from build123d import *

# Parameters (mm, degrees)
SKETCH1_R             = 3.4
SKETCH1_R_2           = 1.9
BOSS_EXTRUDE1_DEPTH   = 5
SKETCH1_R_3           = 14
SKETCH1_R_4           = 10
BOSS_EXTRUDE1_2_DEPTH = 5
BOSS_EXTRUDE3_START   = -5
BOSS_EXTRUDE3_DEPTH   = 5
CUT_EXTRUDE1_DEPTH    = 21.420577857


with BuildPart() as part:
    # Sketch1 → Boss-Extrude1 (new body)
    with BuildSketch(Plane.XY):
        Circle(SKETCH1_R)
        Circle(SKETCH1_R_2, mode=Mode.SUBTRACT)
    extrude(amount=BOSS_EXTRUDE1_DEPTH)



with BuildPart() as body_2:
    # Sketch1 → Boss-Extrude1 2 (new body)
    with BuildSketch(Plane.XY):
        Circle(SKETCH1_R_3)
        Circle(SKETCH1_R_4, mode=Mode.SUBTRACT)
    extrude(amount=BOSS_EXTRUDE1_2_DEPTH)


with BuildPart() as part_1:
    add(part.part)

    add(body_2.part)  # Boss-Extrude3 merges body 2
    # Sketch3 → Boss-Extrude3 (add)
    with BuildSketch(Plane.XY.offset(5).offset(BOSS_EXTRUDE3_START)):
        with BuildLine():
            Line((-2.461082993, -5.681791735), (-1.158545138, -6.104894644))
            ThreePointArc((-1.158545138, -6.104894644), (0.041583332, -6.976727004), (0.5, -8.387490686))
            ThreePointArc((0.5, -8.387490686), (1.026221783, -9.481342425), (2.209302326, -9.752896146))
            ThreePointArc((2.209302326, -9.752896146), (0, -10), (-2.209302326, -9.752896146))
            ThreePointArc((-2.209302326, -9.752896146), (-0.55013353, -8.758786407), (-1.467484664, -7.055976328))
            Line((-1.467484664, -7.055976328), (-2.770022518, -6.632873419))
            ThreePointArc((-2.770022518, -6.632873419), (-4.377477342, -4.842845432), (-3.62455882, -2.557845453))
            ThreePointArc((-3.62455882, -2.557845453), (-3.203111756, -1.874062431), (-3.226850513, -1.071184282))
            ThreePointArc((-3.226850513, -1.071184282), (-2.53927856, -2.260987482), (-1.43690209, -3.081446476))
            ThreePointArc((-1.43690209, -3.081446476), (-3.331173148, -3.837228711), (-2.461082993, -5.681791735))
        make_face()
        with BuildLine():
            Line((-6.164221523, 0.584858813), (-6.164109969, -0.784674291))
            ThreePointArc((-6.164109969, -0.784674291), (-6.622411723, -2.195475308), (-7.822469175, -3.06740542))
            ThreePointArc((-7.822469175, -3.06740542), (-8.700172525, -3.905890853), (-8.592843468, -5.114982027))
            ThreePointArc((-8.592843468, -5.114982027), (-9.510565163, -3.090169944), (-9.958267397, -0.91263928))
            ThreePointArc((-9.958267397, -0.91263928), (-8.500101497, -2.183405771), (-7.164109966, -0.784755745))
            Line((-7.164109966, -0.784755745), (-7.16422152, 0.584777358))
            ThreePointArc((-7.16422152, 0.584777358), (-5.958534597, 2.666706812), (-3.552705858, 2.656742571))
            ThreePointArc((-3.552705858, 2.656742571), (-2.772155254, 2.467223168), (-2.015908439, 2.73790306))
            ThreePointArc((-2.015908439, 2.73790306), (-2.935007106, 1.716313866), (-3.374656916, 0.414355768))
            ThreePointArc((-3.374656916, 0.414355768), (-4.678810484, 1.982365046), (-6.164221523, 0.584858813))
        make_face()
        with BuildLine():
            Line((-1.348615423, 6.04325436), (-2.651084333, 5.619939262))
            ThreePointArc((-2.651084333, 5.619939262), (-4.134458864, 5.619848642), (-5.334551826, 6.491729879))
            ThreePointArc((-5.334551826, 6.491729879), (-6.403224112, 7.067369122), (-7.519971649, 6.591663402))
            ThreePointArc((-7.519971649, 6.591663402), (-5.877852523, 8.090169944), (-3.945245395, 9.188854051))
            ThreePointArc((-3.945245395, 9.188854051), (-4.703218103, 7.409367429), (-2.960178794, 6.570970605))
            Line((-2.960178794, 6.570970605), (-1.657709884, 6.994285702))
            ThreePointArc((-1.657709884, 6.994285702), (0.694900438, 6.490960879), (1.428865848, 4.199802661))
            ThreePointArc((1.428865848, 4.199802661), (1.489825587, 3.398890206), (1.98095058, 2.763301431))
            ThreePointArc((1.98095058, 2.763301431), (0.725344411, 3.321727786), (-0.648750584, 3.337532424))
            ThreePointArc((-0.648750584, 3.337532424), (0.439509241, 5.062397688), (-1.348615423, 6.04325436))
        make_face()
        with BuildLine():
            Line((5.330731354, 3.150077785), (4.525649744, 4.25798777))
            ThreePointArc((4.525649744, 4.25798777), (4.06717562, 5.66873278), (4.525534832, 7.079515131))
            ThreePointArc((4.525534832, 7.079515131), (4.742762387, 8.273765181), (3.945245395, 9.188854051))
            ThreePointArc((3.945245395, 9.188854051), (5.877852523, 8.090169944), (7.519971649, 6.591663402))
            ThreePointArc((7.519971649, 6.591663402), (5.593352853, 6.762646678), (5.334618858, 4.845838918))
            Line((5.334618858, 4.845838918), (6.139700468, 3.737928933))
            ThreePointArc((6.139700468, 3.737928933), (6.388006686, 1.344927632), (4.435793517, -0.06112178))
            ThreePointArc((4.435793517, -0.06112178), (3.692918104, -0.366593497), (3.240203227, -1.030088854))
            ThreePointArc((3.240203227, -1.030088854), (3.383294606, 0.336626808), (2.973707004, 1.648352709))
            ThreePointArc((2.973707004, 1.648352709), (4.950442134, 1.14636879), (5.330731354, 3.150077785))
        make_face()
        with BuildLine():
            Line((4.643188585, -4.096399222), (5.448089696, -2.988358097))
            ThreePointArc((5.448089696, -2.988358097), (6.648111636, -2.116379111), (8.131486169, -2.116348904))
            ThreePointArc((8.131486169, -2.116348904), (9.334412468, -1.953901025), (9.958267397, -0.91263928))
            ThreePointArc((9.958267397, -0.91263928), (9.510565163, -3.090169944), (8.592843468, -5.114982027))
            ThreePointArc((8.592843468, -5.114982027), (8.160100277, -3.229821928), (6.257154566, -3.576077449))
            Line((6.257154566, -3.576077449), (5.452253454, -4.684118574))
            ThreePointArc((5.452253454, -4.684118574), (3.253104814, -5.659749891), (1.312605313, -4.237577998))
            ThreePointArc((1.312605313, -4.237577998), (0.792523319, -3.625457447), (0.021605145, -3.399931355))
            ThreePointArc((0.021605145, -3.399931355), (1.365646649, -3.113680977), (2.486602586, -2.318794424))
            ThreePointArc((2.486602586, -2.318794424), (2.620032257, -4.353902812), (4.643188585, -4.096399222))
        make_face()
    extrude(amount=BOSS_EXTRUDE3_DEPTH)

    # Sketch4 → Cut-Extrude1 (cut, through all)
    with BuildSketch(Plane.XY.offset(5)):
        with BuildLine():
            Line((0.5, -8.387490686), (0.5, -9.387490686))
            ThreePointArc((0.5, -9.387490686), (1.665239053, -10.767667231), (3.221267568, -9.850364333))
            ThreePointArc((3.221267568, -9.850364333), (3.43999971, -9.49227151), (3.786391015, -9.25544397))
            ThreePointArc((3.786391015, -9.25544397), (3.008147158, -9.536826027), (2.209302326, -9.752896146))
            ThreePointArc((2.209302326, -9.752896146), (1.026221783, -9.481342425), (0.5, -8.387490686))
        make_face()
        with BuildLine():
            Line((-0.5, -8.387490686), (-0.5, -9.387490686))
            ThreePointArc((-0.5, -9.387490686), (-1.665239053, -10.767667231), (-3.221267568, -9.850364333))
            ThreePointArc((-3.221267568, -9.850364333), (-3.43999971, -9.49227151), (-3.786391015, -9.25544397))
            ThreePointArc((-3.786391015, -9.25544397), (-3.008147158, -9.536826027), (-2.209302326, -9.752896146))
            ThreePointArc((-2.209302326, -9.752896146), (-1.026221783, -9.481342425), (-0.5, -8.387490686))
        make_face()
        with BuildLine():
            Line((-7.822469175, -3.06740542), (-8.773525691, -3.376422415))
            ThreePointArc((-8.773525691, -3.376422415), (-9.726072919, -4.911128617), (-8.372826765, -6.107537491))
            ThreePointArc((-8.372826765, -6.107537491), (-7.964668303, -6.204907352), (-7.632391128, -6.461161325))
            ThreePointArc((-7.632391128, -6.461161325), (-8.140491944, -5.807959272), (-8.592843468, -5.114982027))
            ThreePointArc((-8.592843468, -5.114982027), (-8.700172525, -3.905890853), (-7.822469175, -3.06740542))
        make_face()
        with BuildLine():
            Line((-8.131486169, -2.116348904), (-9.082542685, -2.425365898))
            ThreePointArc((-9.082542685, -2.425365898), (-10.755247253, -1.743655712), (-10.363679609, 0.019677532))
            ThreePointArc((-10.363679609, 0.019677532), (-10.090705045, 0.338360929), (-9.97250947, 0.740982371))
            ThreePointArc((-9.97250947, 0.740982371), (-9.999629131, -0.086123358), (-9.958267397, -0.91263928))
            ThreePointArc((-9.958267397, -0.91263928), (-9.334412468, -1.953901025), (-8.131486169, -2.116348904))
        make_face()
        with BuildLine():
            Line((-5.334551826, 6.491729879), (-5.922337078, 7.300746873))
            ThreePointArc((-5.922337078, 7.300746873), (-7.676282694, 7.732422823), (-8.395959091, 6.075698576))
            ThreePointArc((-8.395959091, 6.075698576), (-8.36243543, 5.657427869), (-8.503468148, 5.262226664))
            ThreePointArc((-8.503468148, 5.262226664), (-8.039247865, 5.947309792), (-7.519971649, 6.591663402))
            ThreePointArc((-7.519971649, 6.591663402), (-6.403224112, 7.067369122), (-5.334551826, 6.491729879))
        make_face()
        with BuildLine():
            Line((-4.525534832, 7.079515131), (-5.113320084, 7.888532125))
            ThreePointArc((-5.113320084, 7.888532125), (-4.981869307, 9.690028737), (-3.183838679, 9.862525716))
            ThreePointArc((-3.183838679, 9.862525716), (-2.796398978, 9.701390064), (-2.37695879, 9.71339626))
            ThreePointArc((-2.37695879, 9.71339626), (-3.17196352, 9.483598865), (-3.945245395, 9.188854051))
            ThreePointArc((-3.945245395, 9.188854051), (-4.742762387, 8.273765181), (-4.525534832, 7.079515131))
        make_face()
        with BuildLine():
            Line((4.525534832, 7.079515131), (5.113320084, 7.888532125))
            ThreePointArc((5.113320084, 7.888532125), (4.981869307, 9.690028737), (3.183838679, 9.862525716))
            ThreePointArc((3.183838679, 9.862525716), (2.796398978, 9.701390064), (2.37695879, 9.71339626))
            ThreePointArc((2.37695879, 9.71339626), (3.17196352, 9.483598865), (3.945245395, 9.188854051))
            ThreePointArc((3.945245395, 9.188854051), (4.742762387, 8.273765181), (4.525534832, 7.079515131))
        make_face()
        with BuildLine():
            Line((5.334551826, 6.491729879), (5.922337078, 7.300746873))
            ThreePointArc((5.922337078, 7.300746873), (7.676282694, 7.732422823), (8.395959091, 6.075698576))
            ThreePointArc((8.395959091, 6.075698576), (8.36243543, 5.657427869), (8.503468148, 5.262226664))
            ThreePointArc((8.503468148, 5.262226664), (8.039247865, 5.947309792), (7.519971649, 6.591663402))
            ThreePointArc((7.519971649, 6.591663402), (6.403224112, 7.067369122), (5.334551826, 6.491729879))
        make_face()
        with BuildLine():
            Line((8.131486169, -2.116348904), (9.082542685, -2.425365898))
            ThreePointArc((9.082542685, -2.425365898), (10.755247253, -1.743655712), (10.363679609, 0.019677532))
            ThreePointArc((10.363679609, 0.019677532), (10.090705045, 0.338360929), (9.97250947, 0.740982371))
            ThreePointArc((9.97250947, 0.740982371), (9.999629131, -0.086123358), (9.958267397, -0.91263928))
            ThreePointArc((9.958267397, -0.91263928), (9.334412468, -1.953901025), (8.131486169, -2.116348904))
        make_face()
        with BuildLine():
            Line((7.822469175, -3.06740542), (8.773525691, -3.376422415))
            ThreePointArc((8.773525691, -3.376422415), (9.726072919, -4.911128617), (8.372826765, -6.107537491))
            ThreePointArc((8.372826765, -6.107537491), (7.964668303, -6.204907352), (7.632391128, -6.461161325))
            ThreePointArc((7.632391128, -6.461161325), (8.140491944, -5.807959272), (8.592843468, -5.114982027))
            ThreePointArc((8.592843468, -5.114982027), (8.700172525, -3.905890853), (7.822469175, -3.06740542))
        make_face()
    extrude(amount=-CUT_EXTRUDE1_DEPTH, mode=Mode.SUBTRACT)


solid = part_1.part
Verification items for the finished model (mm, model axes). Round coordinates to 2 decimals unless told otherwise and drop trailing zeros. Write each loop counter-clockwise with the first axis right and the second up, starting at its lowest first coordinate (ties: lowest second). Pieces come first, ordered by that corner, then holes.
(1) Material ranges on line 1 (Y direction, x = -9, z = 3.1); line 2 (Y direction, x = -7.75, z = 3.15); line 3 (Y direction, x = 0, z = 3.5), recorded low to high.
Returned:
line 1: y = -10.72 to -5.94, -3.47 to -2.4, 4.36 to 10.72
line 2: y = -11.66 to -6.34, -3.04 to -1.92, 7.69 to 11.66
line 3: y = -14 to -6.92, -3.4 to -1.9, 1.9 to 3.65, 5.77 to 6.93, 10 to 14
(2) Section check A-A (y = 1.25). Enter the section's corners in (x, z), plus the area to 3 significant figures.
Returned:
outline: (-13.94, 0) - (-9.92, 0) - (-9.92, 5) - (-13.94, 5) - close; (-7.07, 0) - (-6, 0) - (-6, 5) - (-7.07, 5) - close; (-3.53, 0) - (-1.43, 0) - (-1.43, 5) - (-3.53, 5) - close; (1.43, 0) - (3.3, 0) - (3.3, 5) - (1.43, 5) - close; (5.09, 0) - (6.34, 0) - (6.34, 5) - (5.09, 5) - close; (9.92, 0) - (13.94, 0) - (13.94, 5) - (9.92, 5) - close
area: 71.7 mm2
(3) Depth check by flat-ended pin: pin 1 Ø1 at (y, z) = (-5.5, 1.5) entering from +X; pin 2 Ø0.8 at (y, z) = (-9, 2.5) entering from -X; pin 3 Ø1.5 at (y, z) = (-8.5, 2.5) entering from +X; pin 4 Ø3 at (x, y) = (-5.5, -2) entering from -Z. Enter the tip coordinate at first touch or a pass-through.
Returned:
pin 1: stops at x = 13.08
pin 2: stops at x = -11.05
pin 3: stops at x = 11.66
pin 4: stops at z = 0
(4) Section check D-D (z = 0.4). Give the number of separate pieces and of enclosed holes in the cut face, plus the area to 3 significant figures.
Returned:
separate pieces: 1
enclosed holes: 6
area: 360 mm2
(5) Section check B-B (x = 7.25). Enter the section's corners in (y, z), plus the area to 3 significant figures.
Returned:
outline: (-11.98, 0) - (-6.89, 0) - (-6.89, 5) - (-11.98, 5) - close; (-3.01, 0) - (-2, 0) - (-2, 5) - (-3.01, 5) - close; (7.86, 0) - (11.98, 0) - (11.98, 5) - (7.86, 5) - close
area: 51.0 mm2
(6) Section check C-C (y = -8). Enter the section's corners in (x, z).
Returned:
outline: (-11.49, 0) - (-6, 0) - (-6, 5) - (-11.49, 5) - close; (-0.55, 0) - (0.47, 0) - (0.47, 5) - (-0.55, 5) - close; (6, 0) - (11.49, 0) - (11.49, 5) - (6, 5) - close
(7) Mould release check, pull along X, two halves, no side actions. Record for faces 1 (the flat face through (0, -3, 0)), 2 (the cylindrical face through (6, -8, 2)): pulls with the +X half, pulls with the -X half, needs draft (parallel to the pull), parting line crosses it, or undercut.
Returned:
face 1: needs draft
face 2: undercut
